Autodesk Inventor part; units mm, degrees
ref_plane "YZ Plane" through (0, 0, 0) normal (1, 0, 0) x (0, 1, 0)
ref_plane "XZ Plane" through (0, 0, 0) normal (0, 1, 0) x (-1, 0, 0)
ref_plane "XY Plane" through (0, 0, 0) normal (0, 0, 1) x (1, 0, 0)
sketch "Sketch3" plane through (0, 0, 0) normal (0, 1, 0) x (-1, 0, 0)
  line L0 (0, 0) -> (0, -2.5)
  line L1 (-1.4434, -2.5) -> (-2.8868, 0)
  line L2 (-2.8868, 0) -> (-1.4434, 2.5)
  line L3 (-1.4434, 2.5) -> (1.4434, 2.5)
  line L4 (1.4434, 2.5) -> (2.8868, 0)
  line L5 (2.8868, 0) -> (1.4434, -2.5)
  line L6 (1.4434, -2.5) -> (-1.4434, -2.5)
  dimension "d3" = 2.5
extrude "Extrusion2" add sketch "Sketch3" along normal blind 10
sketch "Sketch4" plane through (0, 10, 0) normal (0, 1, 0) x (1, 0, 0)
  point P0 (0, 0)
  point P1 (0, 0)
hole "Hole1" at (0, 10, 0) direction (0, -1, 0) diameter 3.6 end through all
properties part number "M3x10"
Read the model definition and answer for the solid it produces. Units are mm, in the model's axes. Coordinates: 2 decimals unless noted, no trailing zeros. Order: outer loops, then holes, each group sorted by start corner. A loop starts at its lowest first (then second) coordinate and runs counter-clockwise, first axis right, second up. Notation, with made-up numbers: (60, 20) - (72, 20) arc R28 cw to (72, 52) - close; hole circle Ø4 at (73, 50.5). An arc over 180 degrees is marked (long way). Answer as a JSON object with one key per item and string values. Group by question number.
Item 1: Consider probe 1 along Z at (x, y) = (0, 3.25); probe 2 along X at (y, z) = (9.75, 1.35); probe 3 along X at (y, z) = (4, -1.2). Determine where each line is inside the solid, lowest interval first. Write a range as from..to.
Item 2: Section B-B (y = 3.5) is taken. Give the vertices of the cut face in (x, z), plus the area to 3 significant figures.
Item 3: Section C-C (z = -0.4) is taken. Give the vertices of the cut face in (x, y) (3 decimals).
Item 4: The mould has two halves that part along X. Classify faces 1 (the face through (-1, 0, 2)), 2 (the face through (-2.175, 4.93, -1.233)), 3 (the face through (-0.541, 4.93, 1.717)): +X half, -X half, draft (parallel to the pull), parting line (faces both ways), or undercut.
Item 5: Section A-A (x = 0) is taken. Give the vertices of the cut face in (y, z).
Item 6: Section D-D (x = 2.1) is taken. Give the vertices of the cut face in (y, z), plus the area to 3 significant figures.
Results are:
{
 "1": {"probe 1": "z = -2.5..-1.8, 1.8..2.5", "probe 2": "x = -2.11..-1.19, 1.19..2.11", "probe 3": "x = -2.19..-1.34, 1.34..2.19"},
 "2": {"outline": "(-2.89, 0) - (-1.44, -2.5) - (1.44, -2.5) - (2.89, 0) - (1.44, 2.5) - (-1.44, 2.5) - close; hole circle Ø3.6 at (0, 0)", "area": "11.5 mm^2"},
 "3": {"outline": "(-2.656, 0) - (-1.755, 0) - (-1.755, 10) - (-2.656, 10) - close; (1.755, 0) - (2.656, 0) - (2.656, 10) - (1.755, 10) - close"},
 "4": {"face 1": "draft", "face 2": "-X half", "face 3": "undercut"},
 "5": {"outline": "(0, -2.5) - (10, -2.5) - (10, -1.8) - (0, -1.8) - close; (0, 1.8) - (10, 1.8) - (10, 2.5) - (0, 2.5) - close"},
 "6": {"outline": "(0, -1.36) - (10, -1.36) - (10, 1.36) - (0, 1.36) - close", "area": "27.3 mm^2"}
}
